Geometry: see drawing. Coordinates: mm, zero at the bounding-box minimum. A direction names the side the tool comes from. Round coordinates to 2 decimals unless told otherwise and drop trailing zeros. Write each loop counter-clockwise with the first axis right and the second up, starting at its lowest first coordinate (ties: lowest second). Pieces come first, ordered by that corner, then holes. Notation, with made-up numbers: M -33,4.5 L -2,4.5 A30 cw -2,40.5 Z; hole C -1,-4 d5. An arc over 180 degrees is marked long. Use one line per item in the form item = value. Start each with the question number.
Item 1: Section query C-C (z = 17). Return loops of the section in (x, y), and give its area (3 significant figures).
Item 2: Section query A-A (y = 25). Return loops of the section in (x, z).
Item 3: Pull-direction query (Z, two-part tool) for the marked faces 1, 2 and 3; classes: pulls with the +Z half, pulls with the -Z half, needs draft (parallel to the pull), parting line crosses it, or undercut.
Item 4: Reachability of the marked faces 4 and 5 from +Z, -Z, +X, -X, +Y, -Y: full face, straight path, thin tool, end or side. Return the list, or none.
Item 5: Ray query, probe 1 along X at (y, z) = (24.5, 6.25); probe 2 along Z at (x, y) = (36.5, 10); probe 3 along Z at (x, y) = (2, 21.5). Return the intervals inside material, ascending.
Item 6: Section query D-D (x = 6). Return loops of the section in (y, z) (3 decimals).
Item 7: Pin query (flat end, axial travel): pin 1 Ø5 at (y, z) = (9.5, 7) entering from +X; pin 2 Ø1.5 at (y, z) = (15.5, 5.5) entering from +X; pin 3 Ø3 at (x, y) = (25, 5) entering from +Z. Return the tip coordinate at first contact, or that it passes through.
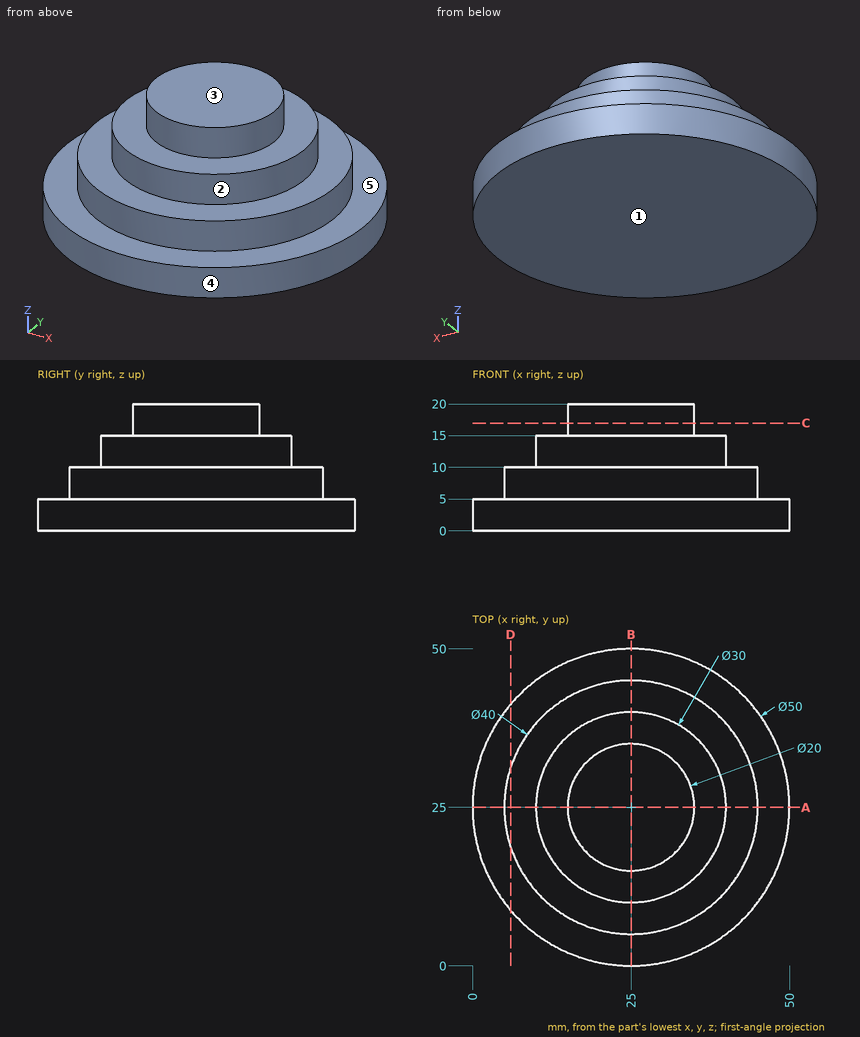
Working result:
q1.outline = C 25,25 d20
q1.area = 314 mm²
q2.outline = M 0,0 L 50,0 L 50,5 L 45,5 L 45,10 L 40,10 L 40,15 L 35,15 L 35,20 L 15,20 L 15,15 L 10,15 L 10,10 L 5,10 L 5,5 L 0,5 Z
q3.face_1 = pulls with the -Z half
q3.face_2 = needs draft
q3.face_3 = pulls with the +Z half
q4.face_4 = +Z, -Z
q4.face_5 = +Z
q5.probe_1 = 5.01 to 44.99
q5.probe_2 = 0 to 10
q5.probe_3 = 0 to 5
q6.outline = M 8.752,0 L 41.248,0 L 41.248,5 L 31.245,5 L 31.245,10 L 18.755,10 L 18.755,5 L 8.752,5 Z
q7.pin_1 = 45.71
q7.pin_2 = 48.35
q7.pin_3 = 10
